from build123d import *

# Parameters (mm, degrees)
F1_DEPTH      = 3
F2_R          = 0.75
F3_DEPTH      = 0.75
F4_R          = 0.75
F5_DEPTH      = 0.75
F6_R          = 0.75
F7_DEPTH      = 25
F8_R          = 1.49999
F9_W          = 8.1852182662
F9_H          = 2.1034856807
F10_DEPTH     = 2.8
F11_R         = 1.5
F13_DEPTH     = 0.5
F14_R         = 0.74999
F15_T1_DEPTH  = 16.1687540342
F15_T6_DEPTH  = 19.9187540342
F15_T11_DEPTH = 19.9187540342
F15_T17_DEPTH = 19.9187540342
F16_R         = 1.49999


# Not quite as in the source:
# - a fillet or chamfer that OpenCascade refuses, or shapes differently, is made with other operations: its cross-section is extruded or revolved along the edge and cut away or added
# - a fillet or chamfer is up to 0.001 mm smaller than in the source, because OpenCascade refuses the exact size
# - a feature names something its author has since deleted; it is built from what else it names


with BuildPart() as f1:
    # F0 (on Top) → F1 (new body)
    with BuildSketch(Plane.XY):
        Polygon((0, 16.1687540342), (0, 0), (7.8920411056, 0), (11.8920411056, 0), (11.8920411056, 16.1687540342), (7.8920411056, 16.1687540342), align=None)
        Polygon((7.8920411056, 19.412382182), (7.8920411056, 16.1687540342), (11.8920411056, 16.1687540342), (15.8920411056, 16.1687540342), (15.8920411056, 19.412382182), align=None)
        Polygon((11.8920411056, 0), (7.8920411056, 0), (7.8920411056, -3.2436281478), (15.8920411056, -3.2436281478), (15.8920411056, 0), align=None)
    extrude(amount=F1_DEPTH)

    # F2 (on face) → F3 (join)
    with BuildSketch(Plane.XZ.offset(-16.1687540342)):
        with Locations((14.8920411056, 1.5)):
            Circle(F2_R)
    extrude(amount=F3_DEPTH)

    # F4 (on face) → F5 (join)
    with BuildSketch(Plane(origin=(0, 0, 0), x_dir=(-1, 0, 0), z_dir=(0, 1, 0))):
        with Locations((-14.8920411056, 1.5)):
            Circle(F4_R)
    extrude(amount=F5_DEPTH)

    # F6 (on face) → F7 (cut)
    with BuildSketch(Plane.XZ):
        with Locations((1.6622071853, 1.5)):
            Circle(F6_R)
    extrude(amount=-F7_DEPTH, mode=Mode.SUBTRACT)

    # F8 (radius 1.5 in the source; OpenCascade refuses exactly that, so slightly less here)
    f8_edges = [f1.edges().sort_by_distance(p)[0] for p in [
        (0, 8.084377, 3),
        (0, 8.084377, 0),
        (15.892041, 17.790568, 3),
        (15.892041, 17.790568, 0),
        (15.892041, -1.621814, 3),
        (15.892041, -1.621814, 0),
    ]]
    fillet(f8_edges, radius=F8_R)

    # F9 (on face) → F10 (join)
    with BuildSketch(Plane.XY.offset(3)):
        with Locations((6.5418113065, 8.0843770171)):
            Rectangle(F9_W, F9_H)
    extrude(amount=F10_DEPTH)

    # F11
    f11_edges = [f1.edges().sort_by_distance(p)[0] for p in [
        (10.63442, 8.084377, 5.8),
        (2.449202, 8.084377, 5.8),
    ]]
    fillet(f11_edges, radius=F11_R)

    # F12 (on face) → F13 (cut)
    with BuildSketch(Plane(origin=(0, 0, 0), x_dir=(1, 0, 0), z_dir=(0, 0, -1))):
        Polygon((5.4570450447, -1.8034656052), (2.8651286848, -8.0843770171), (5.4570450447, -14.365288429), (6.276931148, -14.365288429), (3.6494208034, -8.0843770171), (6.276931148, -1.8034656052), align=None)
        Polygon((7.7570450447, -1.8034656052), (5.1651286848, -8.0843770171), (7.7570450447, -14.365288429), (8.576931148, -14.365288429), (5.9494208034, -8.0843770171), (8.576931148, -1.8034656052), align=None)
    extrude(amount=-F13_DEPTH, mode=Mode.SUBTRACT)

    # F14 (radius 0.75 in the source; OpenCascade refuses exactly that, so slightly less here)
    f14_edges = [f1.edges().sort_by_distance(p)[0] for p in [
        (15.642041, 0.75, 1.5),
        (14.142041, 15.418754, 1.5),
    ]]
    fillet(f14_edges, radius=F14_R)

    # F15: fillet of radius 1.5 on 2 edges, made by hand

    # F15_s2 → F15_t1 (cut)
    with BuildSketch(Plane.XZ.offset(-16.1687540342)):
        with BuildLine():
            ThreePointArc((10.3920411056, 0), (11.4527012774, 0.4393398282), (11.8920411056, 1.5))
            Line((11.8920411056, 1.5), (11.8920411056, 0))
            Line((11.8920411056, 0), (10.3920411056, 0))
        make_face()
    extrude(amount=F15_T1_DEPTH, mode=Mode.SUBTRACT)


with BuildPart() as f15_tool4:
    # F15_s5 → F15_t6 (new body)
    with BuildSketch(Plane.XZ):
        with BuildLine():
            ThreePointArc((10.3920411056, 3), (11.4527012774, 2.5606601718), (11.8920411056, 1.5))
            Line((11.8920411056, 1.5), (11.8920411056, 3))
            Line((11.8920411056, 3), (10.3920411056, 3))
        make_face()
    extrude(amount=-F15_T6_DEPTH)

    split(bisect_by=Plane.XZ.offset(-7.0326341767), keep=Keep.TOP)


with BuildPart() as f1_1:
    add(f1.part)

    # F15_t3: cut F15_tool4
    add(f15_tool4.part, mode=Mode.SUBTRACT)


with BuildPart() as f15_tool9:
    # F15_s10 → F15_t11 (new body)
    with BuildSketch(Plane.XZ.offset(3.75)):
        with BuildLine():
            ThreePointArc((10.3920411056, 3), (11.4527012774, 2.5606601718), (11.8920411056, 1.5))
            Line((11.8920411056, 1.5), (11.8920411056, 3))
            Line((11.8920411056, 3), (10.3920411056, 3))
        make_face()
    extrude(amount=-F15_T11_DEPTH)

    split(bisect_by=Plane.XZ.offset(-7.0326341767), keep=Keep.BOTTOM)

    split(bisect_by=Plane.YZ.offset(10.6344204396), keep=Keep.TOP)


with BuildPart() as f1_2:
    add(f1_1.part)

    # F15_t8: cut F15_tool9
    add(f15_tool9.part, mode=Mode.SUBTRACT)


with BuildPart() as f15_tool15:
    # F15_s16 → F15_t17 (new body)
    with BuildSketch(Plane.XZ.offset(3.75)):
        with BuildLine():
            ThreePointArc((10.3920411056, 3), (11.4527012774, 2.5606601718), (11.8920411056, 1.5))
            Line((11.8920411056, 1.5), (11.8920411056, 3))
            Line((11.8920411056, 3), (10.3920411056, 3))
        make_face()
    extrude(amount=-F15_T17_DEPTH)

    split(bisect_by=Plane.XZ.offset(-9.1361198574), keep=Keep.BOTTOM)


with BuildPart() as f1_3:
    add(f1_2.part)

    # F15_t14: cut F15_tool15
    add(f15_tool15.part, mode=Mode.SUBTRACT)

    # F16 (radius 1.5 in the source; OpenCascade refuses exactly that, so slightly less here)
    f16_edges = [f1_3.edges().sort_by_distance(p)[0] for p in [
        (7.892041, -1.621814, 3),
        (7.892041, -1.621814, 0),
        (7.892041, 17.790568, 3),
        (7.892041, 17.790568, 0),
    ]]
    fillet(f16_edges, radius=F16_R)


solid = f1_3.part
Part model, mm, in its own coordinate system. A direction names the side the tool comes from. Coordinates: 2 decimals unless noted, no trailing zeros. Order: outer loops, then holes, each group sorted by start corner. A loop starts at its lowest first (then second) coordinate and runs counter-clockwise, first axis right, second up.
(1) Slice it at C-C, the plane z = 3.25. Write the cut outline in (x, y).
Check sheet entries:
outline: (2.45, 7.03) - (10.63, 7.03) - (10.63, 9.14) - (2.45, 9.14) - close
(2) Tool access for faces 4 (the face through (4.945, 4.988, 0.246)), 5 (the face through (13, 0, 1)), 6 (the face through (8.32, 17.77, 0.45)): list every direction of +Z, -Z, +X, -X, +Y, -Y with a clear straight run to the whole face (end or side of a thin tool).
Check sheet entries:
face 4: -Z
face 5: none
face 6: -Z, -X, +Y
(3) Pull direction Y, two halves, no side cores. Call faces 1 (the face through (15.441, 17.813, 0.428)), 2 (the face through (5, 0, 1)), 3 (the face through (6.443, 11.181, 0.246)): pulls with the +Y half, pulls with the -Y half, needs draft (parallel to the pull), parting line crosses it, or undercut.
Check sheet entries:
face 1: needs draft
face 2: pulls with the -Y half
face 3: undercut
(4) Pin check, flat tips, straight feed: pin 1 Ø1.5 at (y, z) = (10, 3.5) entering from -X; pin 2 Ø1.5 at (x, z) = (2.5, 1.5) entering from -Y; pin 3 Ø0.6 at (x, z) = (6, 0.5) entering from +Y. Stop position of each tip, or through.
Check sheet entries:
pin 1: stops at x = 0.67
pin 2: stops at y = 0
pin 3: stops at y = 16.17
(5) Probe L1, parallel to Z at x = 6, y = 3.5; L2, parallel to Y at x = 5.5, z = 2.55; L3, parallel to Y at x = 10.5, z = 4.8. List the from-to ranges inside material, lowest first.
Check sheet entries:
L1: z = 0 to 3
L2: y = 0 to 16.17
L3: y = 7.03 to 9.14
